```python
from build123d import *

# Parameters (mm, degrees)
SKETCH1_R           = 90
BOSS_EXTRUDE1_DEPTH = 50
SKETCH2_R           = 50
CUT_EXTRUDE1_DEPTH  = 33.5
SKETCH3_R           = 20
CUT_EXTRUDE2_DEPTH  = 35
SKETCH4_R           = 4
CUT_EXTRUDE3_DEPTH  = 72


with BuildPart() as part:
    # Sketch1 → Boss-Extrude1 (new body)
    with BuildSketch(Plane(origin=(0, 0, 0), x_dir=(1, 0, 0), z_dir=(0, 1, 0))):
        with Locations(Location((0, 0, 0), (0, 0, 270))):
            Circle(SKETCH1_R)
    extrude(amount=BOSS_EXTRUDE1_DEPTH)

    # Sketch2 → Cut-Extrude1 (cut)
    with BuildSketch(Plane(origin=(0, 50, 0), x_dir=(1, 0, 0), z_dir=(0, 1, 0))):
        with Locations(Location((0, 0, 0), (0, 0, 270))):
            Circle(SKETCH2_R)
    extrude(amount=-CUT_EXTRUDE1_DEPTH, mode=Mode.SUBTRACT)

    # Sketch3 → Cut-Extrude2 (cut)
    with BuildSketch(Plane(origin=(0, 16.5, 0), x_dir=(1, 0, 0), z_dir=(0, 1, 0))):
        with Locations(Location((0, 0, 0), (0, 0, 270))):
            Circle(SKETCH3_R)
    extrude(amount=-CUT_EXTRUDE2_DEPTH, mode=Mode.SUBTRACT)

    # Sketch4 → Cut-Extrude3 (cut)
    with BuildSketch(Plane.XZ):
        with Locations(Location((-37.889173801, 12.822266129, 0), (0, 0, 270))):
            Circle(SKETCH4_R)
        with Locations(Location((7.840178699, -39.224120105, 0), (0, 0, 270))):
            Circle(SKETCH4_R)
        with Locations(Location((30.048995102, 26.401853976, 0), (0, 0, 270))):
            Circle(SKETCH4_R)
    extrude(amount=-CUT_EXTRUDE3_DEPTH, mode=Mode.SUBTRACT)


solid = part.part
```
The model under review builds one solid part; all positions refer to its coordinate system, in mm. A direction names the side the tool comes from. Round coordinates to 2 decimals unless told otherwise and drop trailing zeros. Loops run counter-clockwise (first coordinate to the right, second up) from the corner with the lowest first, then second, coordinate; pieces in that order, holes last. Notation, with made-up numbers: (-4, 9.25) -> (35, 9.25) arc R24 ccw to (35, 45.25) -> close; hole circle Ø9 at (69, 33). An arc over 180 degrees is marked (long way). Answer in a Markdown table with one row per item.
1) Tool access review of faces 4 (the cylindrical face through (-19.524, 8.366, -4.336)), 5 (the cylindrical face through (15.02, 33.48, 47.69)): name each direction out of +Z, -Z, +X, -X, +Y, -Y from which nothing blocks a thin tool from reaching the whole face with its end or side.
Taken from the geometry:
| item | result |
|---|---|
| face 4 | +Y, -Y |
| face 5 | +Y |
2) Consider section A-A, the plane z = 0. Write out the cut boundary in (x, y).
Taken from the geometry:
| item | result |
|---|---|
| outline | (-90, 0) -> (-20, 0) -> (-20, 16.5) -> (-50, 16.5) -> (-50, 50) -> (-90, 50) -> close; (20, 0) -> (90, 0) -> (90, 50) -> (50, 50) -> (50, 16.5) -> (20, 16.5) -> close |
3) Consider section B-B, the plane x = 0. Write out the cut boundary in (y, z), plus the area to 3 significant figures.
Taken from the geometry:
| item | result |
|---|---|
| outline | (0, -90) -> (50, -90) -> (50, -50) -> (16.5, -50) -> (16.5, -20) -> (0, -20) -> close; (0, 20) -> (16.5, 20) -> (16.5, 50) -> (50, 50) -> (50, 90) -> (0, 90) -> close |
| area | 4,990 mm² |
4) Consider section C-C, the plane y = 25.5. Write out the cut boundary in (x, z), plus the area to 3 significant figures.
Taken from the geometry:
| item | result |
|---|---|
| outline | circle Ø180 at (0, 0); hole circle Ø100 at (0, 0) |
| area | 17,600 mm² |
5) For pin 1 Ø10 at (y, z) = (33.5, -18) entering from -X; pin 2 Ø10.5 at (x, z) = (-37.89, 12.82) entering from -Y; pin 3 Ø1 at (y, z) = (19.5, 26) entering from -X; pin 4 Ø1.5 at (x, y) = (-35, 6.5) entering from +Z, all flat-tipped, find the tip position at first contact; note any pin that passes through.
Taken from the geometry:
| item | result |
|---|---|
| pin 1 | stops at x = -89.06 |
| pin 2 | stops at y = 0 |
| pin 3 | stops at x = -86.31 |
| pin 4 | stops at z = 83.23 |
6) Consider section D-D, the plane x = 47. Write out the cut boundary in (y, z).
Taken from the geometry:
| item | result |
|---|---|
| outline | (0, -76.75) -> (50, -76.75) -> (50, -17.06) -> (16.5, -17.06) -> (16.5, 17.06) -> (50, 17.06) -> (50, 76.75) -> (0, 76.75) -> close |
7) Wall thickness on line 1 along X through (y, z) = (35, -0.5); line 2 along X through (y, z) = (7.75, 0); line 3 along Z through (x, y) = (18.5, 47): over which ranges is each line inside the solid? List them lowest first.
Taken from the geometry:
| item | result |
|---|---|
| line 1 | x = -90 to -50, 50 to 90 |
| line 2 | x = -90 to -20, 20 to 90 |
| line 3 | z = -88.08 to -46.45, 46.45 to 88.08 |
8) Draft analysis for pull direction Z (two halves, no side actions). For faces 1 (the cylindrical face through (-34.471, 24.65, 83.137)), 2 (the flat face through (-22, 16.5, -1)), 3 (the flat face through (21, 0, -1)), state which applies: pulls with the +Z half, pulls with the -Z half, needs draft (parallel to the pull), parting line crosses it, or undercut.
Taken from the geometry:
| item | result |
|---|---|
| face 1 | parting line crosses it |
| face 2 | undercut |
| face 3 | needs draft |
